```python
from build123d import *

# Parameters (mm, degrees)
SKETCH005_R                = 2
PAD001_DEPTH               = 8
SKETCH006_W                = 10
SKETCH006_H                = 23
POCKET003_DEPTH            = 13.501
POCKET003_DEPTH_BACK       = 13.501
SKETCH007_R                = 2.5
POCKET004_DEPTH            = 12.001
PAD002_DEPTH               = 3.5
PAD002_MIRRORED007_2_DEPTH = 3.5


with BuildPart() as part:
    # Sketch005 → Pad001 (new body)
    with BuildSketch(Plane.YZ):
        with BuildLine():
            ThreePointArc((13.5, 0), (11.174748, 7.574629), (5, 12.539936))
            Line((5, 16.5), (5, 12.539936))
            Line((-5, 16.5), (5, 16.5))
            Line((-5, 12.539936), (-5, 16.5))
            ThreePointArc((-5, 12.539936), (-13.484297, 0.650951), (-6.184658, -12))
            Line((13.5, -12), (-6.184658, -12))
            Line((13.5, 0), (13.5, -12))
        make_face()
        Circle(SKETCH005_R, mode=Mode.SUBTRACT)
    pad001 = extrude(amount=PAD001_DEPTH)

    # Mirrored006: Pad001 across YZ
    add(pad001.mirror(Plane.YZ))

    # Sketch006 → Pocket003 (cut, two sides)
    with BuildSketch(Plane.XZ) as pocket003_sk:
        with Locations((0, 1.5)):
            Rectangle(SKETCH006_W, SKETCH006_H)
    extrude(amount=-POCKET003_DEPTH, mode=Mode.SUBTRACT)
    extrude(pocket003_sk.sketch, amount=POCKET003_DEPTH_BACK, mode=Mode.SUBTRACT)

    # Sketch007 → Pocket004 (cut, through all)
    with BuildSketch(Plane.XY):
        with Locations((0, 9)):
            Circle(SKETCH007_R)
    extrude(amount=-POCKET004_DEPTH, mode=Mode.SUBTRACT)

    # Sketch008 → Pad002 (join)
    with BuildSketch(Plane.XY.offset(13)):
        with BuildLine():
            Line((13.7, 5), (0, 5))
            Line((0, 5), (0, 0))
            Line((0, 0), (8, 0))
            Line((8, 0), (12, 0))
            ThreePointArc((15.4, 0), (13.7, 1.7), (12, 0))
            Line((15.4, 0), (18.7, 0))
            ThreePointArc((18.7, 0), (17.235534, 3.535534), (13.7, 5))
        make_face()
    pad002 = extrude(amount=PAD002_DEPTH)

    # Sketch008 Mirrored007 2 → Pad002 Mirrored007 2 (add)
    with BuildSketch(Plane(origin=(0, 0, 13), x_dir=(-1, 0, 0), z_dir=(0, 0, -1))):
        with BuildLine():
            Line((13.7, 5), (0, 5))
            Line((0, 5), (0, 0))
            Line((0, 0), (8, 0))
            Line((8, 0), (12, 0))
            ThreePointArc((15.4, 0), (13.7, 1.7), (12, 0))
            Line((15.4, 0), (18.7, 0))
            ThreePointArc((18.7, 0), (17.235534, 3.535534), (13.7, 5))
        make_face()
    pad002_mirrored007_2 = extrude(amount=-PAD002_MIRRORED007_2_DEPTH)

    # Mirrored008: Pad002, Pad002 Mirrored007 2 across Sketch008 H_Axis
    add(pad002.mirror(Plane(origin=(0, 0, 13), x_dir=(0, 0, 1), z_dir=(0, 1, 0))))
    add(pad002_mirrored007_2.mirror(Plane(origin=(0, 0, 13), x_dir=(0, 0, 1), z_dir=(0, 1, 0))))


solid = part.part
```
Design review of the part built by this model. Coordinates are the model's own, in mm. A direction names the side the tool comes from. Give positions to 0.01 mm unless a question says otherwise; leave off trailing zeros. Write each loop counter-clockwise with the first axis right and the second up, starting at its lowest first coordinate (ties: lowest second). Pieces come first, ordered by that corner, then holes.
(1) Mouldability with a two-part tool opening along Y and no side actions: class faces 4 (the face through (-0.54, 6.56, -10.99)), 5 (the face through (-5, 3, 1)), 6 (the face through (0, -5, 14)) as +Y half, -Y half, draft (parallel to the pull), parting line (faces both ways), or undercut.
Checked values:
face 4: undercut
face 5: draft
face 6: -Y half
(2) Clearance check with flat-ended pins moving along their axes: pin 1 Ø1.2 at (x, z) = (2.5, 13.5) entering from -Y; pin 2 Ø11.5 at (y, z) = (-3, 5.5) entering from +X; pin 3 Ø2 at (x, y) = (-4.5, -7.5) entering from +Z; pin 4 Ø2.5 at (y, z) = (0, 0) entering from +X. State where each tip first meets the part, or that it passes through.
Checked values:
pin 1: stops at y = -5
pin 2: stops at x = 8
pin 3: stops at z = 11.76
pin 4: passes through
(3) Tool access review of faces 1 (the face through (0, 0, 13)), 2 (the face through (12, -1, 13)), 3 (the face through (-12, -1, 13)): name each direction out of +Z, -Z, +X, -X, +Y, -Y from which nothing blocks a thin tool from reaching the whole face with its end or side.
Checked values:
face 1: +Y, -Y
face 2: -Z, +X, +Y, -Y
face 3: -Z, -X, +Y, -Y
(4) Add section B-B (z = -5). Give the boundary of the cut face in (x, y).
Checked values:
outline: (-8, -12.54) - (-5, -12.54) - (-5, 13.5) - (-8, 13.5) - close; (5, -12.54) - (8, -12.54) - (8, 13.5) - (5, 13.5) - close
(5) Add section A-A (x = -1.5). Give the boundary of the cut face in (y, z), and give its area (3 significant figures).
Checked values:
outline: (-9.07, -10) arc R13.5 ccw to (-6.18, -12) - (7, -12) - (7, -10) - close; (-5, 13) - (5, 13) - (5, 16.5) - (-5, 16.5) - close; (11, -12) - (13.5, -12) - (13.5, -10) - (11, -10) - close
area: 69.5 mm2
(6) Wall thickness on line 1 along X through (y, z) = (7, 6.5); line 2 along Z through (x, y) = (0.5, -2); line 3 along Y through (x, z) = (-5.7, 0): over which ranges is each line inside the solid? List them lowest first.
Checked values:
line 1: x = -8 to -5, 5 to 8
line 2: z = -12 to -10, 13 to 16.5
line 3: y = -13.5 to -2, 2 to 13.5
(7) Add section C-C (y = 7). Give the boundary of the cut face in (x, z), and give its area (3 significant figures).
Checked values:
outline: (-8, -12) - (-1.5, -12) - (-1.5, -10) - (-5, -10) - (-5, 11.54) - (-8, 11.54) - close; (1.5, -12) - (8, -12) - (8, 11.54) - (5, 11.54) - (5, -10) - (1.5, -10) - close
area: 155 mm2
(8) Add section D-D (x = 6). Give the boundary of the cut face in (y, z), and give its area (3 significant figures).
Checked values:
outline: (-6.18, -12) - (13.5, -12) - (13.5, 0) arc R13.5 ccw to (5, 12.54) - (5, 16.5) - (-5, 16.5) - (-5, 12.54) arc R13.5 ccw to start; hole circle Ø4 at (0, 0)
area: 606 mm2
